Could you check a few things on this model? Use its own coordinates, in mm. Face numbers are marked on the shaded views. A direction names the side the tool comes from. Round coordinates to 2 decimals unless told otherwise and drop trailing zeros. Loops run counter-clockwise (first coordinate to the right, second up) from the corner with the lowest first, then second, coordinate; pieces in that order, holes last. Notation, with made-up numbers: (62, 45.5) -> (73, 45.5) arc R3 ccw to (73, 49.5) -> close; hole circle Ø9 at (18, -36.5). An arc over 180 degrees is marked (long way). Write each question's results on one line, items separated by ' | '.
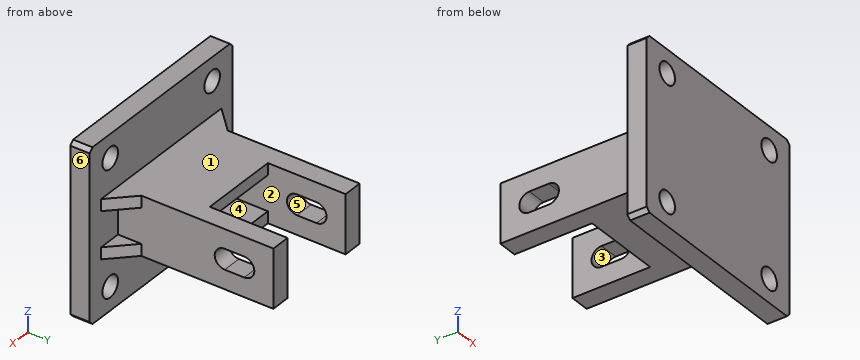
from build123d import *

# Parameters (mm, degrees)
SKETCH1_W           = 50.5
SKETCH1_H           = 44
SKETCH1_R           = 2.75
BOSS_EXTRUDE1_DEPTH = 5
BOSS_EXTRUDE2_START = -14.5
SKETCH3_W           = 5
SKETCH3_H           = 40
BOSS_EXTRUDE2_DEPTH = 15
CUT_EXTRUDE1_REACH  = 66.415
SKETCH5_W           = 20.5
SKETCH5_H           = 20
BOSS_EXTRUDE3_DEPTH = 3
CHAMFER2_SIZE       = 1


with BuildPart() as part:
    # Sketch1 → Boss-Extrude1 (new body)
    with BuildSketch(Plane(origin=(0, 0, 0), x_dir=(1, 0, 0), z_dir=(0, 1, 0))):
        Rectangle(SKETCH1_W, SKETCH1_H)
        with Locations(Location((-18, 16, 0), (0, 0, 270))):
            Circle(SKETCH1_R, mode=Mode.SUBTRACT)
        with Locations(Location((18, 16, 0), (0, 0, 270))):
            Circle(SKETCH1_R, mode=Mode.SUBTRACT)
        with Locations(Location((18, -16, 0), (0, 0, 270))):
            Circle(SKETCH1_R, mode=Mode.SUBTRACT)
        with Locations(Location((-18, -16, 0), (0, 0, 270))):
            Circle(SKETCH1_R, mode=Mode.SUBTRACT)
    extrude(amount=BOSS_EXTRUDE1_DEPTH)

    # Sketch3 → Boss-Extrude2 (add)
    with BuildSketch(Plane.XY.offset(22).offset(BOSS_EXTRUDE2_START)):
        with Locations((-12.75, 25)):
            Rectangle(SKETCH3_W, SKETCH3_H)
        with Locations((12.75, 25)):
            Rectangle(SKETCH3_W, SKETCH3_H)
    extrude(amount=-BOSS_EXTRUDE2_DEPTH)

    # Cut-Extrude1: up to this face of the body (flat: up to its plane)
    cut_extrude1_end = Plane(part.part.faces().sort_by_distance((-15.25, 25, 0))[0])
    # Sketch4 → Cut-Extrude1 (cut, up to the picked face)
    with BuildSketch(Plane(origin=(15.25, 0, 0), x_dir=(0, 0, -1), z_dir=(1, 0, 0)), mode=Mode.PRIVATE) as cut_extrude1_sk1:
        with BuildLine():
            Line((2.6, 37.5), (2.6, 32.5))
            ThreePointArc((2.6, 32.5), (0, 29.9), (-2.6, 32.5))
            Line((-2.6, 32.5), (-2.6, 37.5))
            ThreePointArc((-2.6, 37.5), (0, 40.1), (2.6, 37.5))
        make_face()
    cut_extrude1_tool1 = split(extrude(cut_extrude1_sk1.sketch, amount=-CUT_EXTRUDE1_REACH, mode=Mode.PRIVATE), bisect_by=cut_extrude1_end, keep=Keep.BOTH, mode=Mode.PRIVATE)
    add(cut_extrude1_tool1.solids().sort_by(Axis((15.25, 35, 0), (-1, 0, 0)))[0], mode=Mode.SUBTRACT)

    # Sketch5 → Boss-Extrude3 (add)
    with BuildSketch(Plane.XY.offset(7.5)):
        Polygon((15.25, 11), (21.25, 5), (15.25, 5), align=None)
        Polygon((-21.25, 5), (-15.25, 5), (-15.25, 11), align=None)
        with Locations((0, 15)):
            Rectangle(SKETCH5_W, SKETCH5_H)
    boss_extrude3 = extrude(amount=-BOSS_EXTRUDE3_DEPTH)

    # Mirror1: Boss-Extrude3 across plane
    add(boss_extrude3.mirror(Plane(origin=(0, 0, 0), x_dir=(1, 0, 0), z_dir=(0, 0, -1))))

    # Chamfer2
    chamfer2_edges = [part.edges().sort_by_distance(p)[0] for p in [
        (25.25, 2.5, 22),
        (-25.25, 2.5, 22),
        (-25.25, 2.5, -22),
        (25.25, 2.5, -22),
    ]]
    chamfer(chamfer2_edges, length=CHAMFER2_SIZE)


solid = part.part
1) I want a section at A-A, the plane y = 6.5. Write out the boundary of the cut face in (x, z).
Model answer:
outline: (-19.75, -7.5) -> (19.75, -7.5) -> (19.75, -4.5) -> (15.25, -4.5) -> (15.25, 4.5) -> (19.75, 4.5) -> (19.75, 7.5) -> (-19.75, 7.5) -> (-19.75, 4.5) -> (-15.25, 4.5) -> (-15.25, -4.5) -> (-19.75, -4.5) -> close; hole (-10.25, -4.5) -> (10.25, -4.5) -> (10.25, 4.5) -> (-10.25, 4.5) -> close
2) I want a section at B-B, the plane x = 18. Write out the boundary of the cut face in (y, z).
Model answer:
outline: (0, -22) -> (5, -22) -> (5, -18.75) -> (0, -18.75) -> close; (0, -13.25) -> (5, -13.25) -> (5, -7.5) -> (8.25, -7.5) -> (8.25, -4.5) -> (5, -4.5) -> (5, 4.5) -> (8.25, 4.5) -> (8.25, 7.5) -> (5, 7.5) -> (5, 13.25) -> (0, 13.25) -> close; (0, 18.75) -> (5, 18.75) -> (5, 22) -> (0, 22) -> close
3) For the marked faces 1, 2 and 3, which set-ups out of +Z, -Z, +X, -X, +Y, -Y let a thin tool reach every point of the face, with its end or its side?
Model answer:
face 1: +Z, +X, -X, +Y | face 2: +Y | face 3: +X, -X
4) I'm going to push flat-ended pins straight in: pin 1 (10 mm diameter, centred on x = 1.5, y = 19.5, fed in from +Z); pin 2 (6.5 mm diameter, centred on x = 18, z = 16, fed in from +Y); pin 3 (4.5 mm diameter, centred on x = -18, z = -16, fed in from -Y); pin 4 (6 mm diameter, centred on x = 10.5, y = 15, fed in from -Z). Where does each tip first touch, or does it pass through?
Model answer:
pin 1: stops at z = 7.5 | pin 2: stops at y = 5 | pin 3: passes through | pin 4: stops at z = -7.5
5) I want a section at D-D, the plane y = 31. Write out the boundary of the cut face in (x, z).
Model answer:
outline: (-15.25, -7.5) -> (-10.25, -7.5) -> (-10.25, -2.12) -> (-15.25, -2.12) -> close; (-15.25, 2.12) -> (-10.25, 2.12) -> (-10.25, 7.5) -> (-15.25, 7.5) -> close; (10.25, -7.5) -> (15.25, -7.5) -> (15.25, -2.12) -> (10.25, -2.12) -> close; (10.25, 2.12) -> (15.25, 2.12) -> (15.25, 7.5) -> (10.25, 7.5) -> close
6) I need wall thicknesses on line 1 (X direction, y = 3.75, z = 16); line 2 (Y direction, x = -13, z = 11.5); line 3 (Z direction, x = -10.5, y = 41.5). Which ranges of each line are inside material? Lowest first, please.
Model answer:
line 1: x = -25.25 to -20.75, -15.25 to 15.25, 20.75 to 25.25 | line 2: y = 0 to 5 | line 3: z = -7.5 to 7.5
7) I want a section at C-C, the plane z = 0. Write out the boundary of the cut face in (x, y), plus the area to 4 significant figures.
Model answer:
outline: (-25.25, 0) -> (25.25, 0) -> (25.25, 5) -> (15.25, 5) -> (15.25, 29.9) -> (10.25, 29.9) -> (10.25, 5) -> (-10.25, 5) -> (-10.25, 29.9) -> (-15.25, 29.9) -> (-15.25, 5) -> (-25.25, 5) -> close; (-15.25, 40.1) -> (-10.25, 40.1) -> (-10.25, 45) -> (-15.25, 45) -> close; (10.25, 40.1) -> (15.25, 40.1) -> (15.25, 45) -> (10.25, 45) -> close | area: 550.5 mm2
8) If we mould it in two halves opening along X, with no side actions, what happens to the marked faces 4, 5 and 6? For each: released by +X, released by -X, zero draft, split by the parting line, or undercut.
Model answer:
face 4: undercut | face 5: zero draft | face 6: released by +X
